Model file for the job. Use its own axes, mm. Face numbers are marked on the shaded views. A direction names the side the tool comes from. Give positions to 0.01 mm unless a question says otherwise; leave off trailing zeros. Write each loop counter-clockwise with the first axis right and the second up, starting at its lowest first coordinate (ties: lowest second). Pieces come first, ordered by that corner, then holes.
Autodesk Inventor part; units mm, degrees
ref_plane "YZ Plane" through (0, 0, 0) normal (1, 0, 0) x (0, 1, 0)
ref_plane "XZ Plane" through (0, 0, 0) normal (0, 1, 0) x (-1, 0, 0)
ref_plane "XY Plane" through (0, 0, 0) normal (0, 0, 1) x (1, 0, 0)
sketch "スケッチ1" plane through (0, 0, 0) normal (1, 0, 0) x (0, 1, 0)
  line L0 (0, 0) -> (0, 6)
  line L1 (0, 6) -> (0, -6)
  line L2 (0, 0) -> (11.5, 0)
  line L3 (11.5, 0) -> (11.5, 9.5)
  line L4 (11.5, 9.5) -> (11.5, -9.5)
  circle A0 centre (0, 6) radius 1.25
  circle A1 centre (0, -6) radius 1.25
  circle A2 centre (11.5, 9.5) radius 1.65
  circle A3 centre (11.5, -9.5) radius 1.65
  circle A4 centre (11.5, 9.5) radius 2.5
  circle A5 centre (11.5, -9.5) radius 2.5
  circle A6 centre (0, 0) radius 2.65
  line L5 (0, 0) -> (-14.6, 0)
  circle A7 centre (-14.6, 0) radius 1.65
  circle A8 centre (-14.6, 0) radius 2.5
  circle A9 centre (0, 6) radius 2
  circle A10 centre (0, -6) radius 2
  line L6 (0, 8) -> (10.6499, 11.851)
  line L7 (0, -8) -> (10.6499, -11.851)
  line L8 (-14.6, 0) -> (-14.6, -2.5)
  line L9 (-14.6, 0) -> (-12.1, 0) construction
  line L10 (-14.6, -2.5) -> (-14.6, 2.5)
  line L11 (-14.6, -2.5) -> (-0.7212, -7.8655)
  line L12 (-14.6, 2.5) -> (-0.7212, 7.8655)
  circle A11 centre (11.5, -9.5) radius 14.9164
  line L13 (11.5, -9.5) -> (0, 0)
  line L14 (11.5, -9.5) -> (0, -2.65)
  line L15 (14, 9.5) -> (14, 6.6979)
  circle A12 centre (11.5, -9.5) radius 16.7294
  circle A13 centre (11.5, -9.5) radius 2.6
  circle A14 centre (11.5, -9.5) radius 16.5
  line L16 (14, 6.6979) -> (14.1, -9.4839)
  line L17 (8.9, -9.5) -> (8.9, 0)
  line L18 (9, 9.5) -> (9, 0)
  line L19 (14.0414, 0) -> (11.5, 0)
  line L20 (0, 2.65) -> (2.65, 2.65)
  line L21 (2.65, 2.65) -> (2.65, 0)
  line L22 (2.65, 2.65) -> (2.65, 4.4258)
  point P0 (9.3522, -8.2206)
  point P1 (0, 2.65)
  point P2 (12.4812, 7.2006)
  point P3 (14, 6.8095)
  point P4 (0.3158, 2.6311)
  point P5 (9.2662, -8.1695)
  dimension "d9" = 5
  dimension "d22" = 33
  dimension "d0" = 6
  dimension "d1" = 12
  dimension "d2" = 11.5
  dimension "d3" = 9.5
  dimension "d4" = 19
  dimension "d5" = 2.5
  dimension "d6" = 3.3
  dimension "d7" = 3.3
  dimension "d8" = 5
  dimension "d10" = 5.3
  dimension "d11" = 14.6
  dimension "d12" = 3.3
  dimension "d13" = 5
  dimension "d14" = 4
  dimension "d15" = 4
  dimension "d16" = 90
  dimension "d21" = 5.2
extrude "押し出し3" add sketch "スケッチ1" along normal blind 3 contours A6 L13 L17 L14 | L21 A11 L18 L2 | L2 L17 L13 A6 | L17 L13 A13 L14 | L2 L4 A13 L13 L17 | L21 L22 A14 L18 A11 | L18 A11 L3 L2 | L18 A14 L3 A11 | L19 L16 A13 L4 | L3 A11 L16 L19 | L3 A14 L15 L16 A11
extrude "押し出し4" add sketch "スケッチ1" against normal blind 2 contours L17 L13 A13 L14 | L14 A13 L17 | L2 L4 A13 L13 L17 | A13 L13 A5 L14 | L14 A5 L7 A13 | A13 L4 A5 L13 | L14 A3 L4 A5 | A5 L13 A3 L14 | L7 A5 L4 A13 | L19 L16 A13 L4 | A5 L4 A3 L13
sketch "スケッチ2" plane through (3, 0, 0) normal (1, 0, 0) x (0, 0, -1)
  line L0 (0, 0) -> (0, 11.4707)
  line L1 (0, 14.0414) -> (0, 8.9)
  line L2 (0, 11.4707) -> (-9.5, 11.4707)
  circle A0 centre (-9.5, 11.4707) radius 1.65
  circle A1 centre (-9.5, 11.4707) radius 2.5
  line L3 (-9.5186, 8.9708) -> (0, 8.9)
  line L4 (0, 11.4707) -> (0, 14.0414)
  line L5 (0, 14.0414) -> (-6.6979, 14)
  line L6 (0, 14.0414) -> (-9.5186, 13.9706)
  line L7 (-9.5, 11.4707) -> (-6.8033, 8.9506)
  line L8 (-9.5, 11.4707) -> (-12, 11.4707)
  line L9 (0, 8.9) -> (7.9513, 8.9)
  line L10 (-10.6293, 9.2403) -> (-9.5, 11.4707)
  point P0 (-11.15, 11.4707)
  point P1 (-8.2945, 10.3441)
  point P2 (-10.2453, 9.9986)
  dimension "d27" = 9.5
  dimension "d28" = 3.3
  dimension "d29" = 5
extrude "押し出し5" add sketch "スケッチ2" along normal blind 2 contours L3 L7 A1 L2 L0 | L2 A1 L6 L1 | A1 L7 A0 L2 | L2 A0 L8 A1 | A1 L8 A0 L10
properties part number "ikafly2c2"
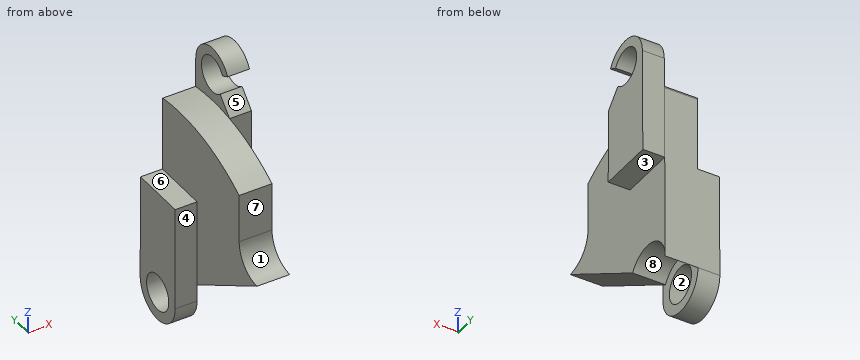
1. Slice it at D-D, the plane y = 9.5. Write the cut outline in (x, z), and give its area (3 significant figures).
Calculated:
outline: (-2, -11.16) - (0, -11.16) - (0, -7.84) - (3, -7.84) - (3, 0) - (5, 0) - (5, 7.39) - (3, 7.39) - (3, 6.88) - (0, 6.88) - (0, 0) - (-2, 0) - close; (3, 10.5) - (5, 10.5) - (5, 11.04) - (3, 11.04) - close
area: 82.3 mm2
2. Slice it at B-B, the plane y = 11.5. Write the cut outline in (x, z), and give its area (3 significant figures).
Calculated:
outline: (-2, -12.1) - (0, -12.1) - (0, -11.15) - (-2, -11.15) - close; (-2, -7.85) - (0, -7.85) - (0, -6.9) - (3, -6.9) - (3, 0) - (5, 0) - (5, 7.85) - (3, 7.85) - (3, 7) - (0, 7) - (0, 0) - (-2, 0) - close; (3, 11.15) - (5, 11.15) - (5, 12) - (3, 12) - close
area: 76.7 mm2
3. Probe probe 1 along Y at (x, z) = (-1.3, -9.5); probe 2 along Z at (x, y) = (-0.85, 11.5); probe 3 along X at (y, z) = (10.75, 5.5). List the from-to ranges inside material, lowest first.
Calculated:
probe 1: y = 8.9 to 9.85, 13.15 to 14.1
probe 2: z = -12.1 to -11.15, -7.85 to 0
probe 3: x = 0 to 5
4. Pull direction Z, two halves, no side cores. Call the marked faces 1, 2 and 3: +Z half, -Z half, draft (parallel to the pull), parting line (faces both ways), or undercut.
Calculated:
face 1: +Z half
face 2: undercut
face 3: -Z half
5. Slice it at A-A, the plane x = -0.5. Write the cut outline in (y, z), and give its area (3 significant figures).
Calculated:
outline: (8.9, -9.5) arc R2.6 ccw (long way) to (14.1, -9.48) - (14.04, 0) - (8.9, 0) - close; hole circle Ø3.3 at (11.5, -9.5)
area: 51.2 mm2
6. Which spindle directions (+Z, -Z, +X, -X, +Y, -Y) get a long thin tool onto all of the face, cutting with end or side? Do the marked faces 4, 5, 6, 7 and 8. Say none if no direction does.
Calculated:
face 4: +Z, -Z, -X, -Y
face 5: +X, -X, -Y
face 6: +Z, -X, +Y, -Y
face 7: +Z, +X, -X, -Y
face 8: -Z, +X
7. Pin check, flat tips, straight feed: P1, Ø5.5, axis at y = 11.5, z = -9.5, coming from the +X side; P2, Ø0.6, axis at x = -1, y = 11.5, coming from the +Z side; P3, Ø1.6, axis at x = -1, z = -5, coming from the -Y side; P4, Ø4, axis at y = 5, z = -8, coming from the -X side. Stop position of each tip, or through.
Calculated:
P1: stops at x = 3
P2: stops at z = 0
P3: stops at y = 8.9
P4: passes through
8. Slice it at C-C, the plane x = 0.75. Write the cut outline in (y, z).
Calculated:
outline: (0, -2.65) - (9.27, -8.17) arc R2.6 cw to (14.1, -9.48) - (14, 6.7) - (14, 6.81) arc R16.5 ccw to (2.65, 4.43) - (2.65, 0) arc R2.65 cw to start
